Verification items for the finished model (mm, model axes). A direction names the side the tool comes from. Give positions to 0.01 mm unless a question says otherwise; leave off trailing zeros. Write each loop counter-clockwise with the first axis right and the second up, starting at its lowest first coordinate (ties: lowest second). Pieces come first, ordered by that corner, then holes. Notation, with made-up numbers: (-31, 68) - (-9, 68) arc R33 cw to (-9, 100) - close; hole circle Ø6 at (22, 6.5). An arc over 180 degrees is marked (long way). Put each result on its own line as item: value.
from build123d import *

# Parameters (mm, degrees)
SKETCH_1_W          = 30
SKETCH_1_H          = 20
EXTRUDE_1_DEPTH     = 5
SKETCH_2_R          = 1.45
CUT_EXTRUDE_1_DEPTH = 19.708286934
SKETCH_3_W          = 15
SKETCH_3_H          = 30
SKETCH_3_R          = 1.45
EXTRUDE_2_DEPTH     = 5
SKETCH_6_W          = 15
SKETCH_6_H          = 5
EXTRUDE_4_DEPTH     = 5
SKETCH_4_R          = 1.45
EXTRUDE_3_DEPTH     = 5
FILLET_2_R          = 1.5


with BuildPart() as part:
    # 草图1 → 凸台-拉伸1 (new body)
    with BuildSketch(Plane(origin=(0, 0, 0), x_dir=(1, 0, 0), z_dir=(0, 1, 0))):
        Rectangle(SKETCH_1_W, SKETCH_1_H)
    extrude(amount=EXTRUDE_1_DEPTH)

    # 草图2 → 切除-拉伸1 (cut, through all)
    with BuildSketch(Plane(origin=(0, 5, 0), x_dir=(1, 0, 0), z_dir=(0, 1, 0))):
        with Locations(Location((-5, 7.5, 0), (0, 0, 270))):
            Circle(SKETCH_2_R)
        with Locations(Location((5, 7.5, 0), (0, 0, 270))):
            Circle(SKETCH_2_R)
        with Locations(Location((5, -7.5, 0), (0, 0, 270))):
            Circle(SKETCH_2_R)
        with Locations(Location((-5, -7.5, 0), (0, 0, 270))):
            Circle(SKETCH_2_R)
    extrude(amount=-CUT_EXTRUDE_1_DEPTH, mode=Mode.SUBTRACT)

    # 草图3 → 凸台-拉伸2 (add)
    # profile 1 of 2: a face of its own
    with BuildSketch(Plane(origin=(0, 5, 0), x_dir=(1, 0, 0), z_dir=(0, 1, 0))):
        with Locations((22.5, 0)):
            Rectangle(SKETCH_3_W, SKETCH_3_H)
        with Locations(Location((22.5, -10, 0), (0, 0, 90))):
            Circle(SKETCH_3_R, mode=Mode.SUBTRACT)
        with Locations(Location((22.5, 10, 0), (0, 0, 90))):
            Circle(SKETCH_3_R, mode=Mode.SUBTRACT)
    # profile 2 of 2: a face of its own
    with BuildSketch(Plane(origin=(0, 5, 0), x_dir=(1, 0, 0), z_dir=(0, 1, 0))):
        with Locations((-22.5, 0)):
            Rectangle(SKETCH_3_W, SKETCH_3_H)
        with Locations(Location((-22.5, 10, 0), (0, 0, 270))):
            Circle(SKETCH_3_R, mode=Mode.SUBTRACT)
        with Locations(Location((-22.5, -10, 0), (0, 0, 270))):
            Circle(SKETCH_3_R, mode=Mode.SUBTRACT)
    extrude(amount=-EXTRUDE_2_DEPTH)

    # 草图6 → 凸台-拉伸4 (add)
    with BuildSketch(Plane(origin=(0, 5, 0), x_dir=(1, 0, 0), z_dir=(0, 1, 0))):
        with Locations((-22.5, -17.5)):
            Rectangle(SKETCH_6_W, SKETCH_6_H)
        with Locations((22.5, -17.5)):
            Rectangle(SKETCH_6_W, SKETCH_6_H)
    extrude(amount=-EXTRUDE_4_DEPTH)

    # 草图4 → 凸台-拉伸3 (add)
    with BuildSketch(Plane(origin=(0, 5, 0), x_dir=(1, 0, 0), z_dir=(0, 1, 0))):
        Polygon((-30, -20), (-75, -20), (-75, -35), (75, -35), (75, -20), (30, -20), (15, -20), (-15, -20), align=None)
        with Locations(Location((-65, -27.5, 0), (0, 0, 270))):
            Circle(SKETCH_4_R, mode=Mode.SUBTRACT)
        with Locations(Location((-22.5, -27.5, 0), (0, 0, 270))):
            Circle(SKETCH_4_R, mode=Mode.SUBTRACT)
        with Locations(Location((22.5, -27.5, 0), (0, 0, 270))):
            Circle(SKETCH_4_R, mode=Mode.SUBTRACT)
        with Locations(Location((65, -27.5, 0), (0, 0, 270))):
            Circle(SKETCH_4_R, mode=Mode.SUBTRACT)
    extrude(amount=-EXTRUDE_3_DEPTH)

    # 圆角2
    fillet_2_edges = [part.edges().sort_by_distance(p)[0] for p in [
        (15, 2.5, -15),
        (30, 2.5, -15),
        (-15, 2.5, -15),
        (-30, 2.5, -15),
        (-15, 2.5, 20),
        (-30, 2.5, 20),
        (15, 2.5, 10),
        (30, 2.5, 20),
        (-15, 2.5, 10),
        (15, 2.5, 20),
        (-15, 2.5, -10),
        (15, 2.5, -10),
        (-75, 2.5, 20),
        (-75, 2.5, 35),
        (75, 2.5, 35),
        (75, 2.5, 20),
    ]]
    fillet(fillet_2_edges, radius=FILLET_2_R)


solid = part.part
Q1. Scan lines: line 1 along X through (y, z) = (3.05, 27.5); line 2 along X through (y, z) = (4.85, 12.5); line 3 along Z through (x, y) = (9.5, 0.8). Record each from-to range of solid material in increasing order.
Answers follow:
line 1: x = -75 to -66.45, -63.55 to -23.95, -21.05 to 21.05, 23.95 to 63.55, 66.45 to 75
line 2: x = -30 to -15, 15 to 30
line 3: z = -10 to 10, 20 to 35
Q2. Go/stop test with flat-tipped pins: pin 1 Ø2.5 at (x, y) = (-58.5, 3.5) entering from -Z; pin 2 Ø3 at (y, z) = (1.5, 10.5) entering from -X; pin 3 Ø2.5 at (x, y) = (-6.5, 2.5) entering from -Z. Record where each tip stops, or that it passes through.
Answers follow:
pin 1: stops at z = 20
pin 2: stops at x = -30
pin 3: stops at z = -10
Q3. Section check B-B, the plane z = 27.5. Record the cut outline in (x, y), plus the area to 3 significant figures.
Answers follow:
outline: (-75, 0) - (-66.45, 0) - (-66.45, 5) - (-75, 5) - close; (-63.55, 0) - (-23.95, 0) - (-23.95, 5) - (-63.55, 5) - close; (-21.05, 0) - (21.05, 0) - (21.05, 5) - (-21.05, 5) - close; (23.95, 0) - (63.55, 0) - (63.55, 5) - (23.95, 5) - close; (66.45, 0) - (75, 0) - (75, 5) - (66.45, 5) - close
area: 692 mm2
Q4. Set-up check for faces 1 (the face through (-1, 5, 21)), 2 (the face through (53, 3, 20)), 3 (the face through (0, 2, 10)): record each of +Z, -Z, +X, -X, +Y, -Y from which the full face is reachable in a straight line by a thin tool's end or side.
Answers follow:
face 1: +Z, -Z, +X, -X, +Y
face 2: -Z, +X, +Y, -Y
face 3: +Y, -Y
Q5. Section check A-A, the plane x = -65. Record the cut outline in (y, z).
Answers follow:
outline: (0, 20) - (5, 20) - (5, 26.05) - (0, 26.05) - close; (0, 28.95) - (5, 28.95) - (5, 35) - (0, 35) - close
Q6. Section check C-C, the plane x = 22.5. Record the cut outline in (y, z).
Answers follow:
outline: (0, -15) - (5, -15) - (5, -11.45) - (0, -11.45) - close; (0, -8.55) - (5, -8.55) - (5, 8.55) - (0, 8.55) - close; (0, 11.45) - (5, 11.45) - (5, 26.05) - (0, 26.05) - close; (0, 28.95) - (5, 28.95) - (5, 35) - (0, 35) - close
Q7. Release check for a two-part mould opening along X. For faces 4 (the face through (23.38, 2.54, 11.15)), 5 (the face through (23.38, 2.54, -8.85)), 6 (the face through (-1, 3, 35)), 7 (the face through (75, 3, 28)) record: released by +X, released by -X, zero draft, split by the parting line, or undercut.
Answers follow:
face 4: undercut
face 5: undercut
face 6: zero draft
face 7: released by +X
Q8. Section check D-D, the plane y = 3.95. Give the number of separate pieces and of enclosed holes in the cut face, plus the area to 3 significant figures.
Answers follow:
separate pieces: 1
enclosed holes: 13
area: 3,820 mm2
